Could you check a few things on this model? Use its own coordinates, in mm. A direction names the side the tool comes from. Coordinates: 2 decimals unless noted, no trailing zeros. Write each loop counter-clockwise with the first axis right and the second up, starting at its lowest first coordinate (ties: lowest second). Pieces come first, ordered by that corner, then holes.
```python
from build123d import *

# Parameters (mm, degrees)
F0_W     = 20.32
F0_H     = 20.32
F1_DEPTH = 2.54
F0_W_2   = 2.54
F0_H_2   = 2.54
F2_DEPTH = 22.86
F3_DEPTH = 25.4
F4_R     = 0.635
F5_DEPTH = 25.4
F6_DEPTH = 20.32


with BuildPart() as f1:
    # F0 (on Top) → F1 (new body)
    with BuildSketch(Plane.XY):
        Rectangle(F0_W, F0_H)
    extrude(amount=F1_DEPTH)

    # F0 (on Top) → F2 (join)
    with BuildSketch(Plane.XY):
        with Locations((-11.43, 0)):
            Rectangle(F0_W_2, F0_H)
        with Locations((-11.43, 11.43)):
            Rectangle(F0_W_2, F0_H_2)
        with Locations((0, 11.43)):
            Rectangle(F0_W, F0_H_2)
        with Locations((11.43, 11.43)):
            Rectangle(F0_W_2, F0_H_2)
        with Locations((11.43, 0)):
            Rectangle(F0_W_2, F0_H)
        with Locations((11.43, -11.43)):
            Rectangle(F0_W_2, F0_H_2)
        with Locations((0, -11.43)):
            Rectangle(F0_W, F0_H_2)
        with Locations((-11.43, -11.43)):
            Rectangle(F0_W_2, F0_H_2)
    extrude(amount=F2_DEPTH)

    # F0 (on Top) → F3 (join)
    with BuildSketch(Plane.XY):
        with Locations((-11.43, -11.43)):
            Rectangle(F0_W_2, F0_H_2)
        with Locations((11.43, -11.43)):
            Rectangle(F0_W_2, F0_H_2)
        with Locations((11.43, 11.43)):
            Rectangle(F0_W_2, F0_H_2)
        with Locations((-11.43, 11.43)):
            Rectangle(F0_W_2, F0_H_2)
    extrude(amount=F3_DEPTH)

    # F4 (on Top) → F5 (cut)
    with BuildSketch(Plane.XY):
        with Locations((-7.62, -11.43)):
            Circle(F4_R)
        with Locations((7.62, -11.43)):
            Circle(F4_R)
        with Locations((11.43, -7.62)):
            Circle(F4_R)
        with Locations((11.43, 7.62)):
            Circle(F4_R)
        with Locations((7.62, 11.43)):
            Circle(F4_R)
        with Locations((-7.62, 11.43)):
            Circle(F4_R)
        with Locations((-11.43, 7.62)):
            Circle(F4_R)
        with Locations((-11.43, -7.62)):
            Circle(F4_R)
    extrude(amount=F5_DEPTH, mode=Mode.SUBTRACT)

    # F0 (on Top) → F6 (join)
    with BuildSketch(Plane.XY):
        with Locations((11.43, -11.43)):
            Rectangle(F0_W_2, F0_H_2)
        with Locations((0, -11.43)):
            Rectangle(F0_W, F0_H_2)
        with Locations((11.43, 0)):
            Rectangle(F0_W_2, F0_H)
        with Locations((-11.43, -11.43)):
            Rectangle(F0_W_2, F0_H_2)
        with Locations((11.43, 11.43)):
            Rectangle(F0_W_2, F0_H_2)
        with Locations((-11.43, 0)):
            Rectangle(F0_W_2, F0_H)
        with Locations((0, 11.43)):
            Rectangle(F0_W, F0_H_2)
        with Locations((-11.43, 11.43)):
            Rectangle(F0_W_2, F0_H_2)
    extrude(amount=F6_DEPTH)


solid = f1.part
```
Item 1: Will these pins go through, and if not, where does the flat tip stop? pin 1 Ø1.4 at (x, y) = (-7.5, 11.5) entering from +Z; pin 2 Ø1.1 at (x, y) = (-11.43, 7.62) entering from +Z; pin 3 Ø6 at (x, y) = (5, 3) entering from +Z; pin 4 Ø5 at (x, y) = (5, -5) entering from -Z.
Item 2: If I drill on line 1 along Y through (x, z) = (11.43, 21) (3 decimals); line 2 along X through (y, z) = (-7.62, 21.95) (3 decimals), over which ranges is the centre line in solid material (lowest first)?
Item 3: If we mould it in two halves opening along Y, with no side actions, what happens to faces 5 (the flat face through (11, -11, 25.4)), 6 (the flat face through (0, 0, 2.54)), 7 (the flat face through (11, -10.16, 24))? For each: released by +Y, released by -Y, zero draft, split by the parting line, or undercut.
Item 4: I want a section at D-D, the plane x = 0.25. List the corners of the cut face in (y, z) for me.
Item 5: I want a section at C-C, the plane y = 11.43. List the corners of the cut face in (x, z) for me (3 decimals), then the cut area to 3 significant figures.
Item 6: I want a section at B-B, the plane z = 13.25. List the corners of the cut face in (x, y) for me, then the cut area to 3 significant figures.
Item 7: Which directions (+Z, -Z, +X, -X, +Y, -Y) give clear straight access to the entire face, cutting with the end or side of a thin tool? Please do faces 1 (the flat face through (0, 0, 0)), 2 (the flat face through (-11, 10.16, 24)), 3 (the flat face through (0, 10.16, 13)), 4 (the flat face through (0, 11, 22.86)).
Item 8: I want a section at A-A, the plane x = -7.62. List the corners of the cut face in (y, z) for me (3 decimals), then the cut area to 3 significant figures.
Taken from the geometry:
1. pin 1: stops at z = 22.86
1. pin 2: stops at z = 20.32
1. pin 3: stops at z = 2.54
1. pin 4: stops at z = 0
2. line 1: y = -12.7 to -8.255, -6.985 to 6.985, 8.255 to 12.7
2. line 2: x = -12.7 to -12.065, -10.795 to -10.16, 10.16 to 10.795, 12.065 to 12.7
3. face 5: zero draft
3. face 6: undercut
3. face 7: undercut
4. outline: (-12.7, 0) - (12.7, 0) - (12.7, 22.86) - (10.16, 22.86) - (10.16, 2.54) - (-10.16, 2.54) - (-10.16, 22.86) - (-12.7, 22.86) - close
5. outline: (-12.7, 0) - (12.7, 0) - (12.7, 25.4) - (10.16, 25.4) - (10.16, 22.86) - (8.255, 22.86) - (8.255, 20.32) - (6.985, 20.32) - (6.985, 22.86) - (-6.985, 22.86) - (-6.985, 20.32) - (-8.255, 20.32) - (-8.255, 22.86) - (-10.16, 22.86) - (-10.16, 25.4) - (-12.7, 25.4) - close
5. area: 587 mm2
6. outline: (-12.7, -12.7) - (12.7, -12.7) - (12.7, 12.7) - (-12.7, 12.7) - close; hole (-10.16, -10.16) - (10.16, -10.16) - (10.16, 10.16) - (-10.16, 10.16) - close
6. area: 232 mm2
7. face 1: -Z, +X, -X, +Y, -Y
7. face 2: +Z, +X, -X
7. face 3: +Z
7. face 4: +Z, +Y, -Y
8. outline: (-12.7, 0) - (12.7, 0) - (12.7, 22.86) - (12.065, 22.86) - (12.065, 20.32) - (10.795, 20.32) - (10.795, 22.86) - (10.16, 22.86) - (10.16, 2.54) - (-10.16, 2.54) - (-10.16, 22.86) - (-10.795, 22.86) - (-10.795, 20.32) - (-12.065, 20.32) - (-12.065, 22.86) - (-12.7, 22.86) - close
8. area: 161 mm2
